Autodesk Fusion 360 part; units mm, degrees
sketch "Sketch1" plane through (0, 0, 0) normal (0, 1, 0) x (1, 0, 0)
  circle A0 centre (0, 0) radius 7.2
  circle A1 centre (0, 0) radius 2.55
  line L0 (7.2, 0) -> (2.55, 0)
  line L1 (2.55, 0) -> (2.55, -28.2)
  line L2 (2.55, -28.2) -> (7.2, -28.2)
  line L3 (7.2, -28.2) -> (7.2, 0)
  line L4 (7.2, -28.2) -> (-3.3, -28.2)
  line L5 (-3.3, -28.2) -> (-3.3, -23.55)
  line L6 (-3.3, -23.55) -> (7.2, -23.55)
  line L7 (7.2, -23.55) -> (7.2, -28.2)
  line L8 (2.55, 0) -> (-7.2, 0)
  line L9 (7.2, -4.2775) -> (7.2, -1.15)
  line L10 (7.2, -14.1) -> (27.0917, -12.0219)
  line L11 (27.0917, -12.0219) -> (26.6179, -7.4866)
  line L12 (26.6179, -7.4866) -> (6.7262, -9.5647)
  line L13 (6.7262, -9.5647) -> (7.2, -14.1)
  line L14 (27.0917, -12.0219) -> (22.58, -10.8963)
  line L15 (22.58, -10.8963) -> (25.0006, -1.1937)
  line L16 (25.0006, -1.1937) -> (29.5123, -2.3192)
  line L17 (29.5123, -2.3192) -> (27.0917, -12.0219)
  dimension "d1" = 14.4
  dimension "d2" = 5.1
  dimension "d3" = 4.65
  dimension "d4" = 28.2
  dimension "d5" = 10.5
  dimension "d6" = 4.65
  dimension "d16" = 20
  dimension "d17" = 4.56
  dimension "d18" = 4.65
  dimension "d19" = 10
extrude "Extrude1" add sketch "Sketch1" along normal blind 4.65 contours A0 A1 L0 L8 | A0 L1 L3 L6 L9 L12 L13 | A0 L0 L1 | L1 L2 L3 L4 L6 L7 | L1 L4 L5 L6 | L3 L10 L12 L14 L15 | L3 L12 L13 | L11 L12 L15 L16 L17 | L11 L12 L14 L15
fillet "Fillet1" radius 2 3 edges at (25.0006, 2.325, 1.1937) (29.5123, 2.325, 2.3192) (27.0917, 2.325, 12.0219)
fillet "Fillet2" radius 2 1 edges at (7.2, 2.325, 28.2)
fillet "Fillet3" radius 2 2 edges at (-0.375, 4.65, 23.55) (-0.375, 0, 23.55)
Read the model definition and answer for the solid it produces. Units are mm, in the model's axes. A direction names the side the tool comes from. Round coordinates to 2 decimals unless told otherwise and drop trailing zeros. Loops run counter-clockwise (first coordinate to the right, second up) from the corner with the lowest first, then second, coordinate; pieces in that order, holes last.
Q1. Each of these flat-tipped pins is pushed along its axis until it touches: pin 1 (1.4 mm diameter, centred on y = 1.5, z = 11, fed in from -X); pin 2 (1.4 mm diameter, centred on y = 2, z = 17.5, fed in from +X). Where does it stop, or does it pass through?
Q2. Which of the six approach directions +Z, -Z, +X, -X, +Y, -Y give full straight-line access (tool end or side, diameter ignored) to faces 1 (the face through (-5, 2, 0)), 2 (the face through (-0.06, 2.29, -2.55)), 3 (the face through (7.2, 2, 5))?
Q3. Section D-D on z = 16.5 is taken. Write down the section's boundary in (x, y), and give its area (3 significant figures).
Q4. Section A-A on x = 1 is taken. Write down the section's boundary in (y, z), and give its area (3 significant figures).
Q5. Determine the mould class of faces 4 (the face through (-0.33, 0.57, 24.15)), 5 (the face through (-3.3, 2, 26)), 6 (the face through (25.45, 2.36, 1.89)) for opening direction X: released by +X, released by -X, zero draft, split by the parting line, or undercut.
Q6. Section B-B on z = -2 is taken. Write down the section's boundary in (x, y), and give its area (3 significant figures).
Q7. Section C-C on y = 0.5 is taken. Write down the section's boundary in (x, z), and give its area (3 significant figures).
Q8. Consider probe 1 along X at (y, z) = (2.45, 25); probe 2 along X at (y, z) = (2.85, 16.5); probe 3 along X at (y, z) = (1.35, -2). Determine where each line is inside the solid, lowest interval first.
Output:
1. pin 1: stops at x = 2.55
1. pin 2: stops at x = 7.2
2. face 1: -X, +Y, -Y
2. face 2: +Y, -Y
2. face 3: -Z, +Y, -Y
3. outline: (2.55, 0) - (7.2, 0) - (7.2, 4.65) - (2.55, 4.65) - close
3. area: 21.6 mm2
4. outline: (0, -7.13) - (4.65, -7.13) - (4.65, -2.35) - (0, -2.35) - close; (0, 25.55) arc R2 ccw to (2, 23.55) - (2.65, 23.55) arc R2 ccw to (4.65, 25.55) - (4.65, 28.2) - (0, 28.2) - close
4. area: 42.2 mm2
5. face 4: zero draft
5. face 5: released by -X
5. face 6: undercut
6. outline: (-6.92, 0) - (-1.58, 0) - (-1.58, 4.65) - (-6.92, 4.65) - close; (1.58, 0) - (6.92, 0) - (6.92, 4.65) - (1.58, 4.65) - close
6. area: 49.6 mm2
7. outline: (-7.2, 0) arc R7.2 ccw to (7.2, 0) - (7.2, 9.52) - (23.35, 7.83) - (24.52, 3.13) arc R2 ccw to (26.94, 1.68) - (27.57, 1.84) arc R2 ccw to (29.03, 4.26) - (27.43, 10.66) arc R2 ccw to (25.7, 12.17) - (7.2, 14.1) - (7.2, 26.2) arc R2 ccw to (5.2, 28.2) - (-3.3, 28.2) - (-3.3, 24.23) - (2.55, 24.23) - (2.55, 0) arc R2.55 cw to (-2.55, 0) - close
7. area: 344 mm2
8. probe 1: x = -3.3 to 7.2
8. probe 2: x = 2.55 to 7.2
8. probe 3: x = -6.92 to -1.58, 1.58 to 6.92
